Part print with two shaded views. Sizes in mm from the minimum x, y, z corner. A direction names the side the tool comes from. Round coordinates to 2 decimals unless told otherwise and drop trailing zeros. Write each loop counter-clockwise with the first axis right and the second up, starting at its lowest first coordinate (ties: lowest second). Pieces come first, ordered by that corner, then holes. Notation, with made-up numbers: M 67,43 L 89,43 A25 ccw 89,68 Z; hole C -31,44 d1. An arc over 180 degrees is marked long. Use one line per item in the form item = value. Start each with the question number.
Item 1: Which spindle directions (+Z, -Z, +X, -X, +Y, -Y) get a long thin tool onto all of the face, cutting with end or side? Do the marked faces 4 and 5. Say none if no direction does.
Item 2: Probe L1, parallel to X at y = 62, z = 35; L2, parallel to Z at x = 78.7, y = 40. List the from-to ranges inside material, lowest first.
Item 3: Cut at C-C, the plane y = 5. Give the cut face in (x, z), then the cut area to 3 significant figures.
Item 4: Cut at D-D, the plane z = 58. Give the cut face in (x, y), then the cut area to 3 significant figures.
Item 5: Flat gauge pin, fed straight in: pin 1 Ø7 at (y, z) = (40, 40) entering from +X. Where does the tip first touch, or does it go through?
Item 6: Mould opens along X. For the marked faces 1, 2 and 3 say: +X half, -X half, draft (parallel to the pull), parting line (faces both ways), or undercut.
Item 7: Cut at B-B, the plane z = 40. Give the cut face in (x, y), then the cut area to 3 significant figures.
Item 8: Cut at A-A, the plane y = 40. Give the cut face in (x, z), then the cut area to 3 significant figures.
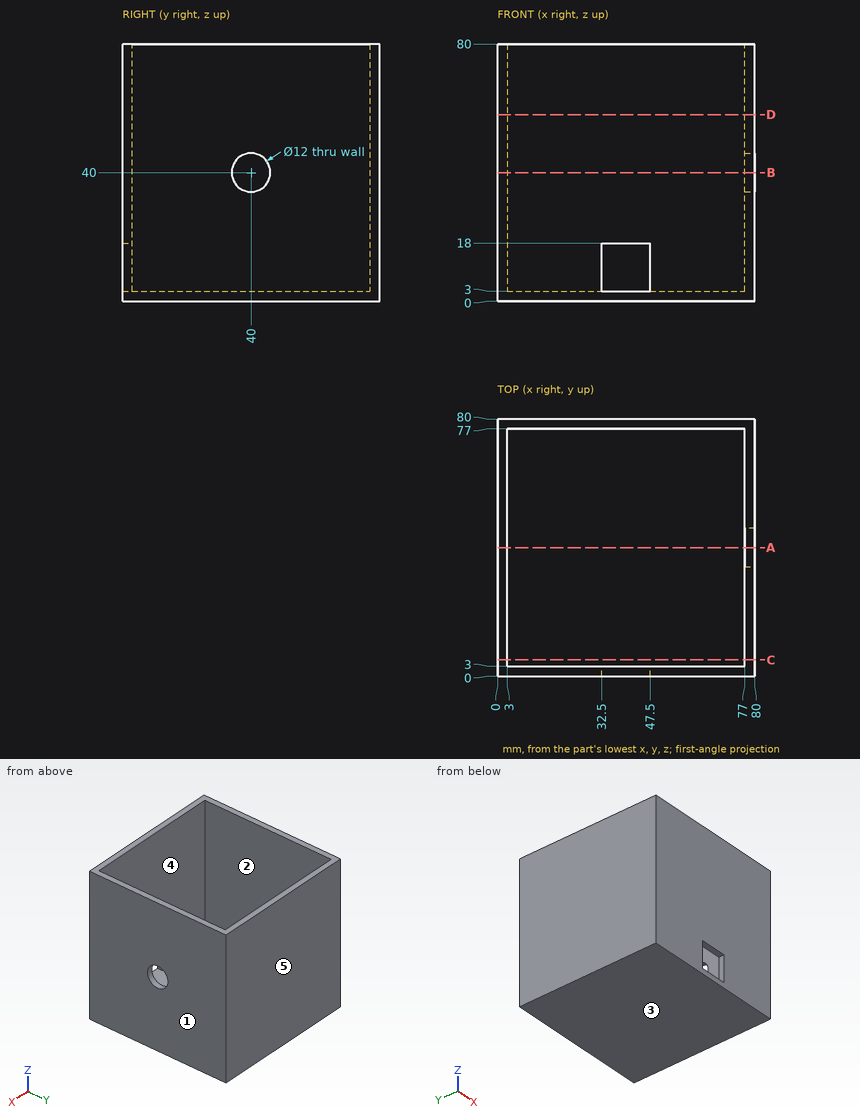
Model answer:
q1.face_4 = +Z
q1.face_5 = +Z, -Z, +X, -X, +Y
q2.L1 = 0 to 3, 77 to 80
q2.L2 = 0 to 34, 46 to 80
q3.outline = M 0,0 L 80,0 L 80,80 L 77,80 L 77,3 L 3,3 L 3,80 L 0,80 Z
q3.area = 702 mm²
q4.outline = M 0,0 L 80,0 L 80,80 L 0,80 Z; hole M 3,3 L 77,3 L 77,77 L 3,77 Z
q4.area = 924 mm²
q5.pin_1 = 3
q6.face_1 = +X half
q6.face_2 = undercut
q6.face_3 = draft
q7.outline = M 0,0 L 80,0 L 80,34 L 77,34 L 77,3 L 3,3 L 3,77 L 77,77 L 77,46 L 80,46 L 80,80 L 0,80 Z
q7.area = 888 mm²
q8.outline = M 0,0 L 80,0 L 80,34 L 77,34 L 77,3 L 3,3 L 3,80 L 0,80 Z; M 77,46 L 80,46 L 80,80 L 77,80 Z
q8.area = 666 mm²
